Part model, mm, in its own coordinate system. Face numbers are marked on the shaded views. Round coordinates to 2 decimals unless told otherwise and drop trailing zeros. Write each loop counter-clockwise with the first axis right and the second up, starting at its lowest first coordinate (ties: lowest second). Pieces come first, ordered by that corner, then holes. Notation, with made-up numbers: M 48,54.5 L 107,54.5 A32 cw 107,86.5 Z; hole C 0.5,67 d10. An arc over 180 degrees is marked long. Answer as a JSON object with one key per item and string values. Group by question number.
1. Band-saw the part on D-D, the plane x = 816. Write the cut outline in (y, z), plus the area to 3 significant figures.
2. Two-plate mould, pull along X, no slides. Class the marked faces 1, 2, 3 and 4: +X half, -X half, draft (parallel to the pull), parting line (faces both ways), or undercut.
3. Band-saw the part on C-C, the plane z = 9.5. Count the separate pieces of the cut face and the enclosed holes in it, plus the area to 3 significant figures.
4. Band-saw the part on B-B, the plane y = -260. Write the cut outline in (x, z), plus the area to 3 significant figures.
5. Band-saw the part on A-A, the plane y = -247.65. Write the cut outline in (x, z), plus the area to 3 significant figures.
6. Drill centre lines: line 1 (X direction, y = -248, z = 11.5); line 2 (X direction, y = -235.5, z = 1.75); line 3 (X direction, y = -237.5, z = 8.5). Where is each one in solid material? Low to high. Write a range as from..to.
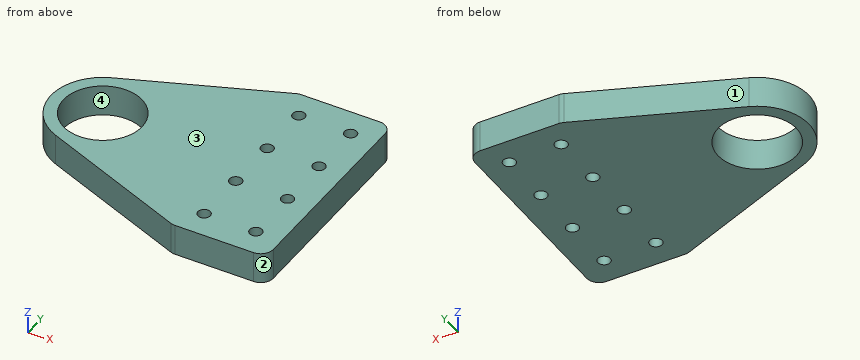
from build123d import *

# Parameters (mm, degrees)
SKETCH1_R           = 16.002
SKETCH1_R_2         = 2.54
BOSS_EXTRUDE1_DEPTH = 12.7


with BuildPart() as part:
    # Sketch1 → Boss-Extrude1 (new body)
    with BuildSketch(Plane.XY):
        with BuildLine():
            Line((877.282099838, -292.1), (909.32, -292.1))
            ThreePointArc((909.32, -292.1), (912.912102448, -290.612102448), (914.4, -287.02))
            Line((914.4, -287.02), (914.4, -208.28))
            ThreePointArc((914.4, -208.28), (912.912102448, -204.687897552), (909.32, -203.2))
            Line((909.32, -203.2), (877.282099838, -203.2))
            ThreePointArc((877.282099838, -203.2), (876.317854156, -203.292352231), (875.388667624, -203.566051077))
            Line((875.388667624, -203.566051077), (814.340256312, -228.087111968))
            ThreePointArc((814.340256312, -228.087111968), (801.116, -247.65), (814.340256312, -267.212888032))
            Line((814.340256312, -267.212888032), (875.388667624, -291.733948923))
            ThreePointArc((875.388667624, -291.733948923), (876.317854156, -292.007647769), (877.282099838, -292.1))
        make_face()
        with Locations((822.198, -247.65)):
            Circle(SKETCH1_R, mode=Mode.SUBTRACT)
        with Locations((903.850524959, -214.298026916)):
            Circle(SKETCH1_R_2, mode=Mode.SUBTRACT)
        with Locations(Location((882.751574878, -214.298026916, 0), (0, 0, 180))):
            Circle(SKETCH1_R_2, mode=Mode.SUBTRACT)
        with Locations((882.751574878, -236.551973084)):
            Circle(SKETCH1_R_2, mode=Mode.SUBTRACT)
        with Locations(Location((903.850524959, -236.551973084, 0), (0, 0, 180))):
            Circle(SKETCH1_R_2, mode=Mode.SUBTRACT)
        with Locations(Location((882.751574878, -258.748026916, 0), (0, 0, 180))):
            Circle(SKETCH1_R_2, mode=Mode.SUBTRACT)
        with Locations((882.751574878, -281.001973084)):
            Circle(SKETCH1_R_2, mode=Mode.SUBTRACT)
        with Locations((903.850524959, -258.748026916)):
            Circle(SKETCH1_R_2, mode=Mode.SUBTRACT)
        with Locations(Location((903.850524959, -281.001973084, 0), (0, 0, 180))):
            Circle(SKETCH1_R_2, mode=Mode.SUBTRACT)
    extrude(amount=BOSS_EXTRUDE1_DEPTH)


solid = part.part
Worked answers:
{
 "1": {"outline": "M -267.88,0 L -262.4,0 L -262.4,12.7 L -267.88,12.7 Z; M -232.9,0 L -227.42,0 L -227.42,12.7 L -232.9,12.7 Z", "area": "139 mm^2"},
 "2": {"face 1": "-X half", "face 2": "+X half", "face 3": "draft", "face 4": "undercut"},
 "3": {"separate pieces": "1", "enclosed holes": "9", "area": "6,750 mm^2"},
 "4": {"outline": "M 805.11,0 L 812.02,0 L 812.02,12.7 L 805.11,12.7 Z; M 832.37,0 L 880.54,0 L 880.54,12.7 L 832.37,12.7 Z; M 884.96,0 L 901.64,0 L 901.64,12.7 L 884.96,12.7 Z; M 906.06,0 L 914.4,0 L 914.4,12.7 L 906.06,12.7 Z", "area": "1,020 mm^2"},
 "5": {"outline": "M 801.12,0 L 806.2,0 L 806.2,12.7 L 801.12,12.7 Z; M 838.2,0 L 914.4,0 L 914.4,12.7 L 838.2,12.7 Z", "area": "1,030 mm^2"},
 "6": {"line 1": "x = 801.12..806.2, 838.2..914.4", "line 2": "x = 804.97..811.78, 832.61..880.44, 885.06..901.54, 906.16..914.4", "line 3": "x = 803.72..809.83, 834.57..880.4, 885.11..901.49, 906.21..914.4"}
}
